Can you work these out from the model? Positions are in its coordinate system, mm. Face numbers are marked on the shaded views. A direction names the side the tool comes from. Round coordinates to 2 decimals unless told otherwise and drop trailing zeros. Loops run counter-clockwise (first coordinate to the right, second up) from the corner with the lowest first, then second, coordinate; pieces in that order, holes last.
(1) If I drill on line 1 along X through (y, z) = (18.5, 0.3); line 2 along Y through (x, z) = (14.75, 2.5); line 3 along X through (y, z) = (8, 1.65), over which ranges is the centre line in solid material (lowest first)?
(2) I want a section at A-A on y = 18. Write out the boundary of the cut face in (x, z), plus the area to 3 significant figures.
(3) I want a section at C-C on x = 15. Write out the boundary of the cut face in (y, z), plus the area to 3 significant figures.
(4) I want a section at B-B on z = 0.55. Write out the boundary of the cut face in (x, y), plus the area to 3 significant figures.
(5) Thinking about a two-plate mould opening in X: for the marked faces 3, 4 and 5, which applies, released by +X, released by -X, zero draft, split by the parting line, or undercut?
(6) Which directions (+Z, -Z, +X, -X, +Y, -Y) give clear straight access to the entire face, cutting with the end or side of a thin tool? Please do the marked faces 1 and 2.
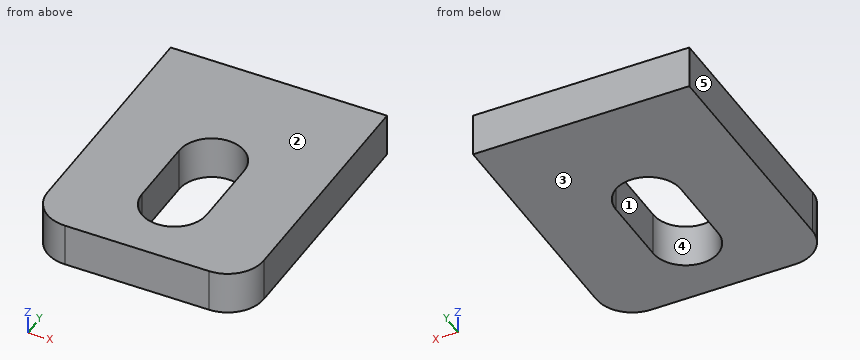
from build123d import *

# Parameters (mm, degrees)
SKETCH_1_W      = 30
SKETCH_1_H      = 38
EXTRUDE_1_DEPTH = 6
FILLET_1_R      = 5


with BuildPart() as part:
    # 草图1 → 凸台-拉伸1 (new body)
    with BuildSketch(Plane.XY):
        with Locations((15, 19)):
            Rectangle(SKETCH_1_W, SKETCH_1_H)
        with BuildLine():
            Line((19.5, 20), (19.5, 10))
            ThreePointArc((19.5, 10), (15, 5.5), (10.5, 10))
            Line((10.5, 10), (10.5, 20))
            ThreePointArc((10.5, 20), (15, 24.5), (19.5, 20))
        make_face(mode=Mode.SUBTRACT)
    extrude(amount=EXTRUDE_1_DEPTH)

    # 圆角1
    fillet_1_edges = [part.edges().sort_by_distance(p)[0] for p in [
        (30, 0, 3),
        (0, 0, 3),
    ]]
    fillet(fillet_1_edges, radius=FILLET_1_R)


solid = part.part
Filled sheet:
1. line 1: x = 0 to 10.5, 19.5 to 30
1. line 2: y = 0 to 5.51, 24.49 to 38
1. line 3: x = 0 to 10.97, 19.03 to 30
2. outline: (0, 0) - (10.5, 0) - (10.5, 6) - (0, 6) - close; (19.5, 0) - (30, 0) - (30, 6) - (19.5, 6) - close
2. area: 126 mm2
3. outline: (0, 0) - (5.5, 0) - (5.5, 6) - (0, 6) - close; (24.5, 0) - (38, 0) - (38, 6) - (24.5, 6) - close
3. area: 114 mm2
4. outline: (0, 5) arc R5 ccw to (5, 0) - (25, 0) arc R5 ccw to (30, 5) - (30, 38) - (0, 38) - close; hole (10.5, 10) arc R4.5 ccw to (19.5, 10) - (19.5, 20) arc R4.5 ccw to (10.5, 20) - close
4. area: 976 mm2
5. face 3: zero draft
5. face 4: undercut
5. face 5: released by -X
6. face 1: +Z, -Z
6. face 2: +Z, +X, -X, +Y, -Y
